Design review of the part built by this model. Coordinates are the model's own, in mm. A direction names the side the tool comes from. Coordinates: 2 decimals unless noted, no trailing zeros. Write each loop counter-clockwise with the first axis right and the second up, starting at its lowest first coordinate (ties: lowest second). Pieces come first, ordered by that corner, then holes. Notation, with made-up numbers: (-31.75, 87) -> (14.25, 87) arc R22 ccw to (14.25, 125) -> close; hole circle Ø6 at (71.5, 1). An arc over 180 degrees is marked (long way). One line per question, with ' | ' between items. Start each with the question number.
Q1. Add section A-A on x = -141. State the section outline as (y, z) points.
Q2. Add section C-C on y = -157.5. State the section outline as (x, z) points.
Q3. Add section B-B on z = 9.5. State the section outline as (x, y) points, and give its area (3 significant figures).
Q4. Wall thickness on probe 1 along X at (y, z) = (77, 6); probe 2 along X at (y, z) = (-96.5, 12.25); probe 3 along Y at (x, z) = (-97, 14.25): over which ranges is each line inside the solid? List them lowest first.
Q5. Draft analysis for pull direction Y (two halves, no side actions). For faces 1 (the flat face through (-93.55, 118.3, 9.93)), 2 (the cylindrical face through (-228.54, -227.53, 9.93)), 3 (the flat face through (118.3, 93.55, 9.93)), 4 (the flat face through (-1, 1, 15)), state which applies: pulls with the +Y half, pulls with the -Y half, needs draft (parallel to the pull), parting line crosses it, or undercut.
Q6. For faces 5 (the flat face through (-118.3, -93.55, 9.93)), 6 (the flat face through (120.96, -96.21, 9.93)), 7 (the flat face through (-96.21, -120.96, 9.93)), list the 3-axis set-ups (+Z, -Z, +X, -X, +Y, -Y) from which the entire face can be reached by the end or side of a thin tool; tool diameter is ignored.
Q7. For P1, Ø1.5, axis at x = -163.5, z = 11.5, coming from the +Y side; P2, Ø12, axis at x = -62, y = 97, coming from the -Z side; P3, Ø1.5, axis at y = -61, z = 6.5, coming from the +X side; P4, Ø5, axis at y = 42, z = 10.5, coming from the +X side, all flat-tipped, find the tip position at first contact; note any pin that passes through.
from build123d import *

# Parameters (mm, degrees)
PAD_DEPTH    = 10
PAD001_DEPTH = 10
PAD002_DEPTH = 10
PAD003_DEPTH = 10
SKETCH002_R  = 22.5
PAD004_DEPTH = 10


with BuildPart() as part:
    # Sketch005 → Pad (new body)
    with BuildSketch(Plane(origin=(0, 0, 5), x_dir=(0, -1, 0), z_dir=(0, 0, 1))):
        Polygon((12.374369, -12.374369), (224.506403, 199.757666), (199.757666, 224.506403), (-12.374369, 12.374369), align=None)
    extrude(amount=PAD_DEPTH)

    # Sketch004 → Pad001 (join)
    with BuildSketch(Plane(origin=(0, 0, 5), x_dir=(-1, 0, 0), z_dir=(0, 0, 1))):
        Polygon((12.374369, -12.374369), (224.506403, 199.757666), (199.757666, 224.506403), (-12.374369, 12.374369), align=None)
    extrude(amount=PAD001_DEPTH)

    # Sketch001 → Pad002 (join)
    with BuildSketch(Plane.XY.offset(5)):
        Polygon((12.374369, -12.374369), (224.506403, 199.757666), (199.757666, 224.506403), (-12.374369, 12.374369), align=None)
    extrude(amount=PAD002_DEPTH)

    # Sketch003 → Pad003 (join)
    with BuildSketch(Plane(origin=(0, 0, 5), x_dir=(0, 1, 0), z_dir=(0, 0, 1))):
        Polygon((12.374369, -12.374369), (224.506403, 199.757666), (199.757666, 224.506403), (-12.374369, 12.374369), align=None)
    extrude(amount=PAD003_DEPTH)

    # Sketch002 → Pad004 (join)
    with BuildSketch(Plane.XY.offset(5)):
        with Locations((212.132034, 212.132034)):
            Circle(SKETCH002_R)
        with Locations((212.132034, -212.132034)):
            Circle(SKETCH002_R)
        with Locations((-212.132034, -212.132034)):
            Circle(SKETCH002_R)
        with Locations((-212.132034, 212.132034)):
            Circle(SKETCH002_R)
    extrude(amount=PAD004_DEPTH)


solid = part.part
Output values:
1) outline: (-165.75, 5) -> (-116.25, 5) -> (-116.25, 15) -> (-165.75, 15) -> close; (116.25, 5) -> (165.75, 5) -> (165.75, 15) -> (116.25, 15) -> close
2) outline: (-182.25, 5) -> (-132.75, 5) -> (-132.75, 15) -> (-182.25, 15) -> close; (132.75, 5) -> (182.25, 5) -> (182.25, 15) -> (132.75, 15) -> close
3) outline: (-214.51, -189.76) arc R22.5 ccw (long way) to (-189.76, -214.51) -> (0, -24.75) -> (189.76, -214.51) arc R22.5 ccw (long way) to (214.51, -189.76) -> (24.75, 0) -> (214.51, 189.76) arc R22.5 ccw (long way) to (189.76, 214.51) -> (0, 24.75) -> (-189.76, 214.51) arc R22.5 ccw (long way) to (-214.51, 189.76) -> (-24.75, 0) -> close | area: 44,300 mm2
4) probe 1: x = -101.75 to -52.25, 52.25 to 101.75 | probe 2: x = -121.25 to -71.75, 71.75 to 121.25 | probe 3: y = -121.75 to -72.25, 72.25 to 121.75
5) face 1: pulls with the +Y half | face 2: undercut | face 3: undercut | face 4: needs draft
6) face 5: +Z, -Z, -X | face 6: +Z, -Z, +X | face 7: +Z, -Z, -Y
7) P1: stops at y = 189 | P2: passes through | P3: stops at x = 86.5 | P4: stops at x = 69.25
